Autodesk Inventor part; units mm, degrees
ref_plane "YZ Plane" through (0, 0, 0) normal (1, 0, 0) x (0, 1, 0)
ref_plane "XZ Plane" through (0, 0, 0) normal (0, 1, 0) x (-1, 0, 0)
ref_plane "XY Plane" through (0, 0, 0) normal (0, 0, 1) x (1, 0, 0)
sketch "Sketch1" plane through (0, 0, 0) normal (1, 0, 0) x (0, 1, 0)
  arc A0 (-10.9904, -24.3236) -> (-10.9904, 33.6895) centre (1.9201, 4.683) ccw
  arc A1 (-36.9675, 40.4029) -> (-10.9904, 33.6895) centre (-19.7566, 53.3848) ccw
  arc A2 (-10.9904, -24.3236) -> (-36.9675, -31.0369) centre (-19.7566, -44.0189) ccw
  line L0 (-36.9675, 40.4029) -> (-36.9675, -31.0369)
  circle A3 centre (1.9201, 4.683) radius 0.9144
  dimension "d1" = 1.8288
extrude "Extrusion1" add sketch "Sketch1" along normal blind 6.35
sketch "Sketch2" plane through (0, -36.9675, -31.0369) normal (0, -1, 0) x (1, 0, 0)
  point P0 (0, 31.0369)
sketch "Sketch3" plane through (0, -36.9675, -31.0369) normal (0, -1, 0) x (1, 0, 0)
  line L0 (6.35, 71.4398) -> (6.35, 62.8637)
  line L1 (0, 71.4398) -> (6.35, 71.4398)
  line L2 (6.35, 71.4398) -> (0, 71.4398)
  line L3 (0, 71.4398) -> (0, 0)
  line L4 (0, 71.4398) -> (0, 0)
  line L5 (0, 0) -> (6.35, 0)
  line L6 (0, 0) -> (6.35, 0)
  line L7 (6.35, 0) -> (6.35, 71.4398)
  point P0 (0, 31.0369)
  point P1 (6.35, 64.7265)
extrude "Extrusion2" add sketch "Sketch3" along normal blind 1.27
properties part number "Base Hinge 2x"
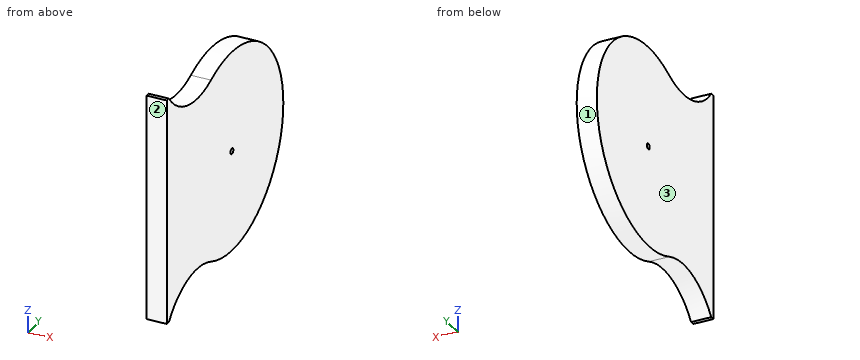
Could you check a few things on this model? Use its own coordinates, in mm. Face numbers are marked on the shaded views. Round coordinates to 2 decimals unless told otherwise and drop trailing zeros. Loops run counter-clockwise (first coordinate to the right, second up) from the corner with the lowest first, then second, coordinate; pieces in that order, holes last. Notation, with made-up numbers: (53.5, -10) - (103.5, -10) arc R26 ccw to (103.5, 24) - close; hole circle Ø3 at (84.5, 35). An arc over 180 degrees is marked (long way). Write item = value, one per line.
1) I need wall thicknesses on line 1 along Y through (x, z) = (0.75, -24.5); line 2 along Z through (x, y) = (1.25, -20.5); line 3 along Z through (x, y) = (1.25, -35). Which ranges of each line are inside material? Lowest first, please. Write a range as from..to.
Computed:
line_1 = -38.24..-28.91, -10.59..14.43
line_2 = -22.47..31.84
line_3 = -28.77..38.14
2) Imagine slicing it at A-A (x = 3). Please give me the cut outline in (y, z).
Computed:
outline = (-38.24, -31.04) - (-36.97, -31.04) arc R21.56 cw to (-10.99, -24.32) arc R31.75 ccw (long way) to (-10.99, 33.69) arc R21.56 cw to (-36.97, 40.4) - (-38.24, 40.4) - close; hole circle Ø1.83 at (1.92, 4.68)
3) If we mould it in two halves opening along Y, with no side actions, what happens to the marked faces 1, 2 and 3? For each: pulls with the +Y half, pulls with the -Y half, needs draft (parallel to the pull), parting line crosses it, or undercut.
Computed:
face_1 = undercut
face_2 = pulls with the -Y half
face_3 = needs draft
4) Imagine slicing it at C-C (z = -8.5). Please give me the cut outline in (x, y).
Computed:
outline = (0, -38.24) - (6.35, -38.24) - (6.35, 30.8) - (0, 30.8) - close
5) Imagine slicing it at B-B (y = -27.5). Please give me the cut outline in (x, z).
Computed:
outline = (0, -23.9) - (6.35, -23.9) - (6.35, 33.27) - (0, 33.27) - close
